For this review, take the finished solid that the model builds, in its own axes (mm). Give positions to 0.01 mm unless a question says otherwise; leave off trailing zeros. Write each loop counter-clockwise with the first axis right and the second up, starting at its lowest first coordinate (ties: lowest second). Pieces come first, ordered by that corner, then holes. Notation, with made-up numbers: (-23.5, 58) -> (-13.5, 58) arc R18 cw to (-13.5, 82) -> close; hole circle Ø4 at (7.5, -5.75). An arc over 180 degrees is marked (long way). Write item = value, one per line.
```python
from build123d import *

# Parameters (mm, degrees)
F1_DEPTH = 12
F2_R     = 3
F3_DEPTH = 12.001


with BuildPart() as f1:
    # F0 (on Front) → F1 (new body)
    with BuildSketch(Plane.XZ):
        Polygon((-30.699901, 0), (-30.699901, -12), (44.300099, -12), (44.300099, -9.5), (14.300099, 0), align=None)
    extrude(amount=F1_DEPTH)

    # F2 (on face) → F3 (cut, through all)
    with BuildSketch(Plane.XY):
        with Locations((-22.699901, -6)):
            Circle(F2_R)
        with Locations((7.300099, -6)):
            Circle(F2_R)
    extrude(amount=-F3_DEPTH, mode=Mode.SUBTRACT)


solid = f1.part
```
(1) Take a section at C-C (z = -10.25). Write out the cut boundary in (x, y).
Answers below:
outline = (-30.7, -12) -> (44.3, -12) -> (44.3, 0) -> (-30.7, 0) -> close; hole circle Ø6 at (-22.7, -6); hole circle Ø6 at (7.3, -6)
(2) Take a section at A-A (y = -6). Write out the cut boundary in (x, z), plus the area to 4 significant figures.
Answers below:
outline = (-30.7, -12) -> (-25.7, -12) -> (-25.7, 0) -> (-30.7, 0) -> close; (-19.7, -12) -> (4.3, -12) -> (4.3, 0) -> (-19.7, 0) -> close; (10.3, -12) -> (44.3, -12) -> (44.3, -9.5) -> (14.3, 0) -> (10.3, 0) -> close
area = 613.5 mm^2
(3) Take a section at B-B (x = 6.5). Write out the cut boundary in (y, z).
Answers below:
outline = (-12, -12) -> (-8.89, -12) -> (-8.89, 0) -> (-12, 0) -> close; (-3.11, -12) -> (0, -12) -> (0, 0) -> (-3.11, 0) -> close
(4) The part is to be moulded in two halves that separate along Y. For faces 1 (the face through (-2, 0, -6)), 2 (the face through (-2, -12, -6)), 3 (the face through (8.91, -3.47, -5.92)), say which applies: released by +Y, released by -Y, zero draft, split by the parting line, or undercut.
Answers below:
face_1 = released by +Y
face_2 = released by -Y
face_3 = undercut
(5) To check wall thickness, follow probe 1 along X at (y, z) = (-3.25, -10.5); probe 2 along X at (y, z) = (-4.25, -10.75); probe 3 along Y at (x, z) = (10, -7). State the ranges of each line that lie inside material, in increasing order.
Answers below:
probe_1 = -30.7 to -23.9, -21.5 to 6.1, 8.5 to 44.3
probe_2 = -30.7 to -25.14, -20.26 to 4.86, 9.74 to 44.3
probe_3 = -12 to -7.31, -4.69 to 0
(6) Take a section at D-D (x = 35.5). Write out the cut boundary in (y, z), plus the area to 3 significant figures.
Answers below:
outline = (-12, -12) -> (0, -12) -> (0, -6.71) -> (-12, -6.71) -> close
area = 63.4 mm^2
